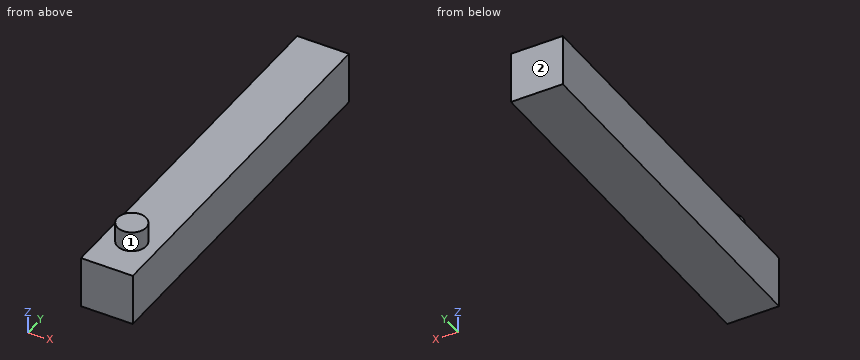
```python
from build123d import *

# Parameters (mm, degrees)
SKETCH1_W           = 65
SKETCH1_H           = 9
BOSS_EXTRUDE1_DEPTH = 6.25
SKETCH3_W           = 9
SKETCH3_H           = 65
SKETCH3_R           = 2.5
CUT_EXTRUDE2_DEPTH  = 3.5


with BuildPart() as part:
    # Sketch1 → Boss-Extrude1 (new, symmetric)
    with BuildSketch(Plane(origin=(0, 0, 0), x_dir=(0, 1, 0), z_dir=(0, 0, 1))):
        Rectangle(SKETCH1_W, SKETCH1_H)
    extrude(amount=BOSS_EXTRUDE1_DEPTH, both=True)

    # Sketch3 → Cut-Extrude2 (cut)
    with BuildSketch(Plane.XY.offset(6.25)):
        Rectangle(SKETCH3_W, SKETCH3_H)
        with Locations((0, -25)):
            Circle(SKETCH3_R, mode=Mode.SUBTRACT)
    extrude(amount=-CUT_EXTRUDE2_DEPTH, mode=Mode.SUBTRACT)


solid = part.part
```
Geometry check sheet. Reference: the model listing, model coordinates, mm. Face numbers are marked on the shaded views. A direction names the side the tool comes from. Give positions to 0.01 mm unless a question says otherwise; leave off trailing zeros. Write each loop counter-clockwise with the first axis right and the second up, starting at its lowest first coordinate (ties: lowest second). Pieces come first, ordered by that corner, then holes. Notation, with made-up numbers: (-5, 81.5) -> (40, 81.5) arc R20 cw to (40, 92.5) -> close; hole circle Ø3 at (48.25, 68). An arc over 180 degrees is marked (long way). Use one line per item in the form item = value.
Item 1: Scan line: line 1 (Z direction, x = -2.25, y = 19). Record every from-to range of solid material in increasing order.
Results list:
line_1 = -6.25 to 2.75
Item 2: Sectioned sample at D-D on y = 28. Enter the section's corners in (x, z).
Results list:
outline = (-4.5, -6.25) -> (4.5, -6.25) -> (4.5, 2.75) -> (-4.5, 2.75) -> close
Item 3: Sectioned sample at A-A on y = -25. Enter the section's corners in (x, z), plus the area to 3 significant figures.
Results list:
outline = (-4.5, -6.25) -> (4.5, -6.25) -> (4.5, 2.75) -> (2.5, 2.75) -> (2.5, 6.25) -> (-2.5, 6.25) -> (-2.5, 2.75) -> (-4.5, 2.75) -> close
area = 98.5 mm2
Item 4: Sectioned sample at C-C on z = 5.5. Enter the section's corners in (x, y), plus the area to 3 significant figures.
Results list:
outline = circle Ø5 at (0, -25)
area = 19.6 mm2
Item 5: Depth check by flat-ended pin: pin 1 Ø1 at (x, z) = (-0.5, 4.5) entering from +Y; pin 2 Ø4 at (x, y) = (0.5, -1) entering from +Z. Enter the tip coordinate at first touch or a pass-through.
Results list:
pin_1 = -22.5
pin_2 = 2.75
Item 6: Access from +Z, -Z, +X, -X, +Y, -Y to the whole of each face (thin tool, end or side, straight path). Record for the marked faces 1 and 2.
Results list:
face_1 = +Z
face_2 = +Z, -Z, +X, -X, +Y
Item 7: Sectioned sample at B-B on x = 0. Enter the section's corners in (y, z).
Results list:
outline = (-32.5, -6.25) -> (32.5, -6.25) -> (32.5, 2.75) -> (-22.5, 2.75) -> (-22.5, 6.25) -> (-27.5, 6.25) -> (-27.5, 2.75) -> (-32.5, 2.75) -> close
